Part model, mm, in its own coordinate system. Give positions to 0.01 mm unless a question says otherwise; leave off trailing zeros. Order: outer loops, then holes, each group sorted by start corner. A loop starts at its lowest first (then second) coordinate and runs counter-clockwise, first axis right, second up. Notation, with made-up numbers: M 63,48.25 L 87,48.25 A24 ccw 87,68.25 Z; hole C 81.5,87 d11. An arc over 180 degrees is marked long. Return JSON: item names as keys, results as strings.
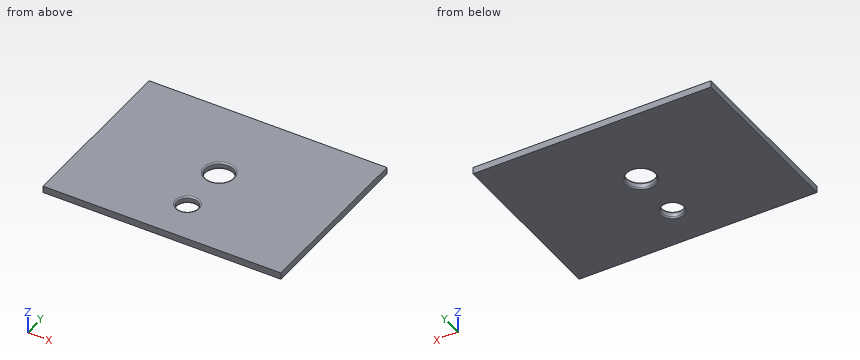
from build123d import *

# Parameters (mm, degrees)
SKETCH1_W           = 169.8
SKETCH1_H           = 125
SKETCH1_R           = 10
BOSS_EXTRUDE1_DEPTH = 4.8
SKETCH2_R           = 7.5
CUT_EXTRUDE1_DEPTH  = 5.8
FILLET1_R           = 1


with BuildPart() as part:
    # Sketch1 → Boss-Extrude1 (new body)
    with BuildSketch(Plane.XY):
        Rectangle(SKETCH1_W, SKETCH1_H)
        with Locations((0, 5)):
            Circle(SKETCH1_R, mode=Mode.SUBTRACT)
    extrude(amount=BOSS_EXTRUDE1_DEPTH)

    # Sketch2 → Cut-Extrude1 (cut, through all)
    with BuildSketch(Plane.XY.offset(4.8)):
        with Locations((0, -32.5)):
            Circle(SKETCH2_R)
    extrude(amount=-CUT_EXTRUDE1_DEPTH, mode=Mode.SUBTRACT)

    # Fillet1
    fillet1_edges = [part.edges().sort_by_distance(p)[0] for p in [
        (-10, 5, 0),
        (-10, 5, 4.8),
        (-7.5, -32.5, 0),
        (-7.5, -32.5, 4.8),
    ]]
    fillet(fillet1_edges, radius=FILLET1_R)


solid = part.part
Q1. Band-saw the part on C-C (z = 1.95). Give the cut face in (x, y).
Established:
{"outline": "M -84.9,-62.5 L 84.9,-62.5 L 84.9,62.5 L -84.9,62.5 Z; hole C 0,5 d20; hole C 0,-32.5 d15"}
Q2. Pin check, flat tip, straight feed: pin 1 (12 mm diameter, centred on x = 0, y = 5, fed in from +Z). Stop position of the tip, or through.
Established:
{"pin 1": "passes through"}
Q3. Band-saw the part on B-B (y = -32.5). Give the cut face in (x, z).
Established:
{"outline": "M -84.9,0 L -8.5,0 A1 ccw -7.5,1 L -7.5,3.8 A1 ccw -8.5,4.8 L -84.9,4.8 Z; M 7.5,1 A1 ccw 8.5,0 L 84.9,0 L 84.9,4.8 L 8.5,4.8 A1 ccw 7.5,3.8 Z"}
Q4. Band-saw the part on A-A (x = 0). Give the cut face in (y, z), then the cut area to 3 significant figures.
Established:
{"outline": "M -62.5,0 L -41,0 A1 ccw -40,1 L -40,3.8 A1 ccw -41,4.8 L -62.5,4.8 Z; M -25,1 A1 ccw -24,0 L -6,0 A1 ccw -5,1 L -5,3.8 A1 ccw -6,4.8 L -24,4.8 A1 ccw -25,3.8 Z; M 15,1 A1 ccw 16,0 L 62.5,0 L 62.5,4.8 L 16,4.8 A1 ccw 15,3.8 Z", "area": "430 mm²"}
Q5. Probe line 1 along X through (y, z) = (-35, 1.4). List the from-to ranges inside material, lowest first.
Established:
{"line 1": "x = -84.9 to -7.07, 7.07 to 84.9"}
Q6. Band-saw the part on D-D (y = 5). Give the cut face in (x, z), then the cut area to 3 significant figures.
Established:
{"outline": "M -84.9,0 L -11,0 A1 ccw -10,1 L -10,3.8 A1 ccw -11,4.8 L -84.9,4.8 Z; M 10,1 A1 ccw 11,0 L 84.9,0 L 84.9,4.8 L 11,4.8 A1 ccw 10,3.8 Z", "area": "718 mm²"}
